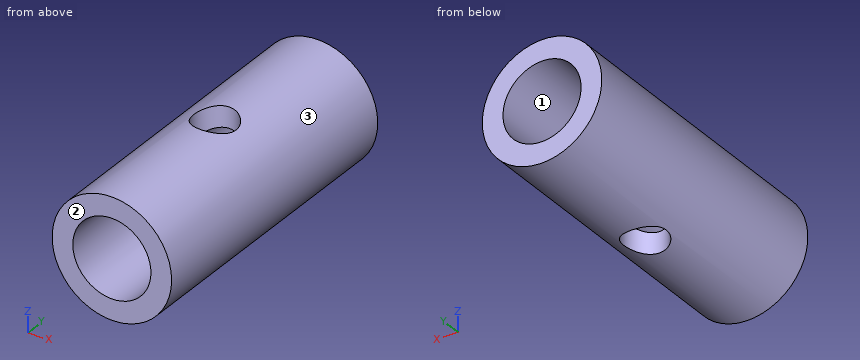
```python
from build123d import *

# Parameters (mm, degrees)
F0_R          = 10
F1_DEPTH      = 50
F2_R          = 3.55
F3_DEPTH      = 25
F3_DEPTH_BACK = 25
F4_R          = 6.5365859356
F5_DEPTH      = 60


with BuildPart() as f1:
    # F0 (on Front) → F1 (new body)
    with BuildSketch(Plane.XZ):
        Circle(F0_R)
    extrude(amount=F1_DEPTH)

    # F2 (on Top) → F3 (cut, two sides)
    with BuildSketch(Plane.XY) as f3_sk:
        with Locations((0, -25)):
            Circle(F2_R)
    extrude(amount=-F3_DEPTH, mode=Mode.SUBTRACT)
    extrude(f3_sk.sketch, amount=F3_DEPTH_BACK, mode=Mode.SUBTRACT)

    # F4 (on face) → F5 (cut)
    with BuildSketch(Plane(origin=(0, 0, 0), x_dir=(-1, 0, 0), z_dir=(0, 1, 0))):
        Circle(F4_R)
    extrude(amount=-F5_DEPTH, mode=Mode.SUBTRACT)


solid = f1.part
```
Geometry: final body of the model. Coordinates: model frame, mm. Face numbers are marked on the shaded views. Coordinates: 2 decimals unless noted, no trailing zeros. Write each loop counter-clockwise with the first axis right and the second up, starting at its lowest first coordinate (ties: lowest second). Pieces come first, ordered by that corner, then holes. Notation, with made-up numbers: M 10,-10 L 47,-10 A21 cw 47,7 Z; hole C 59.5,-31 d11. An arc over 180 degrees is marked long. Use CSV: the item, a comma, the result in double quotes. Start each with the question number.
1. Cut plane B-B on z = 0. Return the cut outline in (x, y).
2. Cut plane D-D on y = -44. Return the cut outline in (x, z).
3. First-contact query: P1, Ø8, axis at y = -43, z = 5.5, coming from the +X side; P2, Ø1.5, axis at x = 6, y = -24.5, coming from the +Z side; P3, Ø1.5, axis at x = -4, y = -16, coming from the +Z side; P4, Ø9, axis at x = 0, y = -25, coming from the -Z side. Flat tips, straight axial feed; report the tip coordinate or a pass-through.
4. Mould query, pull axis X, two halves, no side actions, for the marked faces 1, 2 and 3. Classes: pulls with the +X half, pulls with the -X half, needs draft (parallel to the pull), parting line crosses it, or undercut.
5. Cut plane A-A on x = 0. Return the cut outline in (y, z).
6. Ray query, probe 1 along Y at (x, z) = (0, 6.95); probe 2 along Z at (x, y) = (-5.5, -33.5); probe 3 along Z at (x, y) = (1.75, -33). Return the intervals inside material, ascending.
7. Cut plane C-C on y = -25. Return the cut outline in (x, z), plus the area to 3 significant figures.
Entries:
1,outline,"M -10,-50 L -6.54,-50 L -6.54,0 L -10,0 Z; M 6.54,-50 L 10,-50 L 10,0 L 6.54,0 Z"
2,outline,"C 0,0 d20; hole C 0,0 d13.07"
3,P1,"x = 9.89"
3,P2,"z = 8.51"
3,P3,"z = 9.46"
3,P4,"z = -10"
4,face 1,"undercut"
4,face 2,"needs draft"
4,face 3,"parting line crosses it"
5,outline,"M -50,-10 L -28.55,-10 L -28.55,-6.54 L -50,-6.54 Z; M -50,6.54 L -28.55,6.54 L -28.55,10 L -50,10 Z; M -21.45,-10 L 0,-10 L 0,-6.54 L -21.45,-6.54 Z; M -21.45,6.54 L 0,6.54 L 0,10 L -21.45,10 Z"
6,probe 1,"-50 to -28.55, -21.45 to 0"
6,probe 2,"-8.35 to -3.53, 3.53 to 8.35"
6,probe 3,"-9.85 to -6.3, 6.3 to 9.85"
7,outline,"M -3.55,-9.35 L -3.55,-5.49 A6.54 cw -3.55,5.49 L -3.55,9.35 A10 ccw Z; M 3.55,-9.35 A10 ccw 3.55,9.35 L 3.55,5.49 A6.54 cw 3.55,-5.49 Z"
7,area,"129 mm²"
